Autodesk Inventor part; units mm, degrees
ref_plane "YZ Plane" through (0, 0, 0) normal (1, 0, 0) x (0, 1, 0)
ref_plane "XZ Plane" through (0, 0, 0) normal (0, 1, 0) x (-1, 0, 0)
ref_plane "XY Plane" through (0, 0, 0) normal (0, 0, 1) x (1, 0, 0)
sketch "Sketch1" plane through (0, 0, 0) normal (0, 1, 0) x (-1, 0, 0)
  line L0 (-12.7, -63.5) -> (12.7, -63.5)
  line L1 (12.7, -63.5) -> (12.7, 63.5)
  line L2 (12.7, 63.5) -> (-12.7, 63.5)
  line L3 (-12.7, 63.5) -> (-12.7, -63.5)
  line L4 (-12.7, -63.5) -> (12.7, 63.5) construction
  line L5 (12.7, -63.5) -> (-12.7, 63.5) construction
  point P0 (0, 0)
  dimension "d0" = 25.4
  dimension "d1" = 127
extrude "Plate1" add sketch "Sketch1" along normal blind 3.048
sketch "Sketch2" plane through (-15.748, 6.096, 63.5) normal (-1, 0, 0) x (0, -1, 0)
  line L0 (0, -127) -> (0, 0)
  line L1 (0, 0) -> (-247.904, 0)
  line L2 (-247.904, 0) -> (-247.904, -127)
  line L3 (-247.904, -127) -> (0, -127)
edge flange "Flange1" height 254 angle 90 thickness 3.048 bend radius 3.048 thickness toward (-1, 0, 0) relief tear relief width 3.048 relief depth 1.524 edges at (-12.7, 3.048, 0) wall of the first edge with corners at (-15.748, 6.096, -63.5) (-15.748, 6.096, 63.5) (-15.748, 254, 63.5) (-15.748, 254, -63.5)
bend "Bend1"
corner "Corner1"
sketch "Sketch3" plane through (0, 3.048, 0) normal (0, 1, 0) x (1, 0, 0)
  line L0 (-12.7, 63.5) -> (12.7, 63.5) construction
  line L1 (-12.7, -63.5) -> (-12.7, 63.5) construction
  line L2 (12.7, -63.5) -> (-12.7, -63.5) construction
  line L3 (12.7, 63.5) -> (12.7, -63.5) construction
  line L4 (12.7, 0) -> (-12.7, 0) construction
  point P0 (0, 0)
  point P1 (0, -6.35)
  point P2 (0, 0)
  point P3 (0, -31.75)
  point P4 (0, -57.15)
  point P5 (0, -82.55)
  point P6 (0, -107.95)
  point P7 (0, 6.35)
  point P8 (0, 31.75)
  point P9 (0, 57.15)
  point P10 (0, 82.55)
  point P11 (0, 107.95)
  dimension "d13" = 6.35
  dimension "d16" = 25.4
  dimension "d21" = 12.7
hole "Hole1" at (0, 3.048, 6.35) at (0, 3.048, 31.75) at (0, 3.048, 57.15) at (0, 3.048, 82.55) at (0, 3.048, -82.55) at (0, 3.048, -57.15) at (0, 3.048, -31.75) at (0, 3.048, -6.35) direction (0, -1, 0) diameter 5.1054 end through all
sketch "Sketch4" plane through (-12.7, 257.048, 63.5) normal (0, 1, 0) x (-1, 0, 0)
  line L0 (0, -127) -> (0, 0)
  line L1 (0, 0) -> (-25.4, 0)
  line L2 (-25.4, 0) -> (-25.4, -127)
  line L3 (-25.4, -127) -> (0, -127)
edge flange "Flange2" height 31.496 angle 90 thickness 3.048 bend radius 3.048 thickness toward (0, 1, 0) relief tear relief width 3.048 relief depth 1.524 edges at (-15.748, 254, 0) wall of the first edge with corners at (-12.7, 257.048, -63.5) (-12.7, 257.048, 63.5) (12.7, 257.048, 63.5) (12.7, 257.048, -63.5)
bend "Bend2"
corner "Corner2"
sketch "Sketch5" plane through (12.7, 260.096, 63.5) normal (0, 1, 0) x (1, 0, 0)
  circle A0 centre (-12.7, 6.35) radius 2.5527 construction
  circle A1 centre (-12.7, 31.75) radius 2.5527 construction
  circle A2 centre (-12.7, 57.15) radius 2.5527 construction
  circle A3 centre (-12.7, 69.85) radius 2.5527 construction
  circle A4 centre (-12.7, 95.25) radius 2.5527 construction
  circle A5 centre (-12.7, 120.65) radius 2.5527 construction
  point P0 (-12.7, 63.5)
  point P1 (-12.7, 6.35)
  point P2 (-12.7, 31.75)
  point P3 (-12.7, 57.15)
  point P4 (-12.7, 69.85)
  point P5 (-12.7, 95.25)
  point P6 (-12.7, 120.65)
hole "Hole2" at (0, 260.096, 57.15) at (0, 260.096, 31.75) at (0, 260.096, 6.35) at (0, 260.096, -6.35) at (0, 260.096, -31.75) at (0, 260.096, -57.15) direction (0, -1, 0) diameter 5.1054 end through all
equation "\"d27\" = Thickness"
equation "\"d44\" = Thickness"
equation "\"d2\" = Thickness"
equation "\"d3\" = BendReliefWidth"
equation "\"d4\" = BendReliefDepth"
equation "\"d5\" = MinimumRemnant"
equation "\"d6\" = TransitionRadius"
equation "\"d9\" = BendRadius"
equation "\"d10\" = CornerReliefSize"
equation "\"d11\" = GapSize"
equation "\"d12\" = JacobiRadiusSize"
equation "\"d29\" = BendReliefWidth"
equation "\"d30\" = BendReliefDepth"
equation "\"d31\" = MinimumRemnant"
equation "\"d32\" = TransitionRadius"
equation "\"d35\" = BendRadius"
equation "\"d36\" = CornerReliefSize"
equation "\"d37\" = GapSize"
equation "\"d38\" = JacobiRadiusSize"
equation "\"BendRadius\" = Thickness"
equation "\"BendReliefWidth\" = Thickness"
equation "\"BendReliefDepth\" = 0.5 * Thickness"
equation "\"CornerReliefSize\" = 4 * Thickness"
equation "\"MinimumRemnant\" = 2 * Thickness"
equation "\"TransitionRadius\" = BendRadius"
equation "\"JacobiRadiusSize\" = BendRadius"
equation "\"GapSize\" = Thickness"
properties part number "trough_back_support" material "Aluminum 6061"
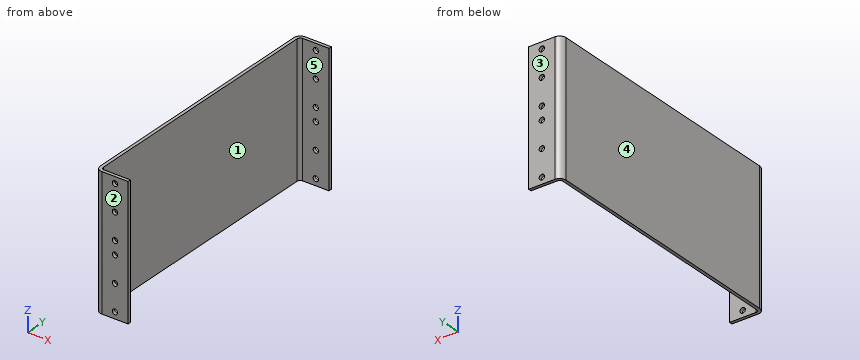
Geometry check sheet. Reference: the model listing, model coordinates, mm. Face numbers are marked on the shaded views. A direction names the side the tool comes from. Coordinates: 2 decimals unless noted, no trailing zeros. Write each loop counter-clockwise with the first axis right and the second up, starting at its lowest first coordinate (ties: lowest second). Pieces come first, ordered by that corner, then holes. Notation, with made-up numbers: M 75,76.25 L 104,76.25 A21 cw 104,107.25 Z; hole C 84,72.5 d4. An arc over 180 degrees is marked long. One line per item, written item: value. Start each with the question number.
(1) Depth check by flat-ended pin: pin 1 (4 mm diameter, centred on x = 0, z = -57.15, fed in from +Y); pin 2 (8 mm diameter, centred on y = 164.5, z = 48, fed in from +X); pin 3 (1.5 mm diameter, centred on x = -14, z = 14.5, fed in from +Y). Enter the tip coordinate at first touch or a pass-through.
(2) Scan lines: line 1 along Y through (x, z) = (11, 39); line 2 along Y through (x, z) = (-13, -3); line 3 along X through (y, z) = (22.5, -9). Record each from-to range of solid material in increasing order. Write a range as [from, to].
(3) Tool access check on the marked faces 4 and 5. Record the directions out of +Z, -Z, +X, -X, +Y, -Y that give a thin tool (end or side, any length) a straight path to the whole face; none if there is none.
(4) Sectioned sample at C-C, the plane z = 0.5. Enter the section's corners in (x, y), and give its area (3 significant figures).
(5) Release check for a two-part mould opening along Y. For the marked faces 1, 2 and 3 record: released by +Y, released by -Y, zero draft, split by the parting line, or undercut.
(6) Sectioned sample at A-A, the plane x = 8. Enter the section's corners in (y, z), and give its area (3 significant figures).
(7) Sectioned sample at D-D, the plane y = 90. Enter the section's corners in (x, z), and give its area (3 significant figures).
(8) Sectioned sample at B-B, the plane z = 31.75. Enter the section's corners in (x, y).
Filled sheet:
1. pin 1: through
1. pin 2: x = -15.75
1. pin 3: y = 260.07
2. line 1: [0, 3.05], [257.05, 260.1]
2. line 2: [0.01, 3.06], [257.03, 260.09]
2. line 3: [-18.8, -15.75]
3. face 4: +Z, -Z, -X, +Y, -Y
3. face 5: +Z, -Z, +X
4. outline: M -18.8,6.1 A6.1 ccw -12.7,0 L 12.7,0 L 12.7,3.05 L -12.7,3.05 A3.05 cw -15.75,6.1 L -15.75,254 A3.05 cw -12.7,257.05 L 12.7,257.05 L 12.7,260.1 L -12.7,260.1 A6.1 ccw -18.8,254 Z
4. area: 954 mm²
5. face 1: undercut
5. face 2: released by -Y
5. face 3: released by +Y
6. outline: M 0,-63.5 L 3.05,-63.5 L 3.05,63.5 L 0,63.5 Z; M 257.05,-63.5 L 260.1,-63.5 L 260.1,63.5 L 257.05,63.5 Z
6. area: 774 mm²
7. outline: M -18.8,-63.5 L -15.75,-63.5 L -15.75,63.5 L -18.8,63.5 Z
7. area: 387 mm²
8. outline: M -18.8,6.1 A6.1 ccw -12.7,0 L -2.55,0 L -2.55,3.05 L -12.7,3.05 A3.05 cw -15.75,6.1 L -15.75,254 A3.05 cw -12.7,257.05 L -2.55,257.05 L -2.55,260.1 L -12.7,260.1 A6.1 ccw -18.8,254 Z; M 2.55,0 L 12.7,0 L 12.7,3.05 L 2.55,3.05 Z; M 2.55,257.05 L 12.7,257.05 L 12.7,260.1 L 2.55,260.1 Z
